Check sheet for the drawn part. Datum: minimum x, y, z corner. Units: mm. Coordinates: 2 decimals unless noted, no trailing zeros. Order: outer loops, then holes, each group sorted by start corner. A loop starts at its lowest first (then second) coordinate and runs counter-clockwise, first axis right, second up. Notation, with made-up numbers: M 62,66.5 L 94,66.5 A20 cw 94,105.5 Z; hole C 10,62 d11. An arc over 180 degrees is marked long. Return JSON: item names as keys, results as strings. Group by question number.
Q1. Section check C-C, the plane z = 1.1. Enter the section's corners in (x, y) (1 decimal), then the cut area to 3 significant figures.
Q2. Section check B-B, the plane x = 24.3. Count the separate pieces of the cut face and the enclosed holes in it, then the cut area to 3 significant figures.
Q3. Section check A-A, the plane y = 3. Enter the section's corners in (x, z).
Q4. Thickness scan on probe 1 along Y at (x, z) = (24.3, 0.3); probe 2 along X at (y, z) = (37.5, 0.5); probe 3 along X at (y, z) = (41.5, 1.25) (1 decimal). Record the ranges inside material, lowest first.
Q5. Section check D-D, the plane y = 40.31. Enter the section's corners in (x, z), then the cut area to 3 significant figures.
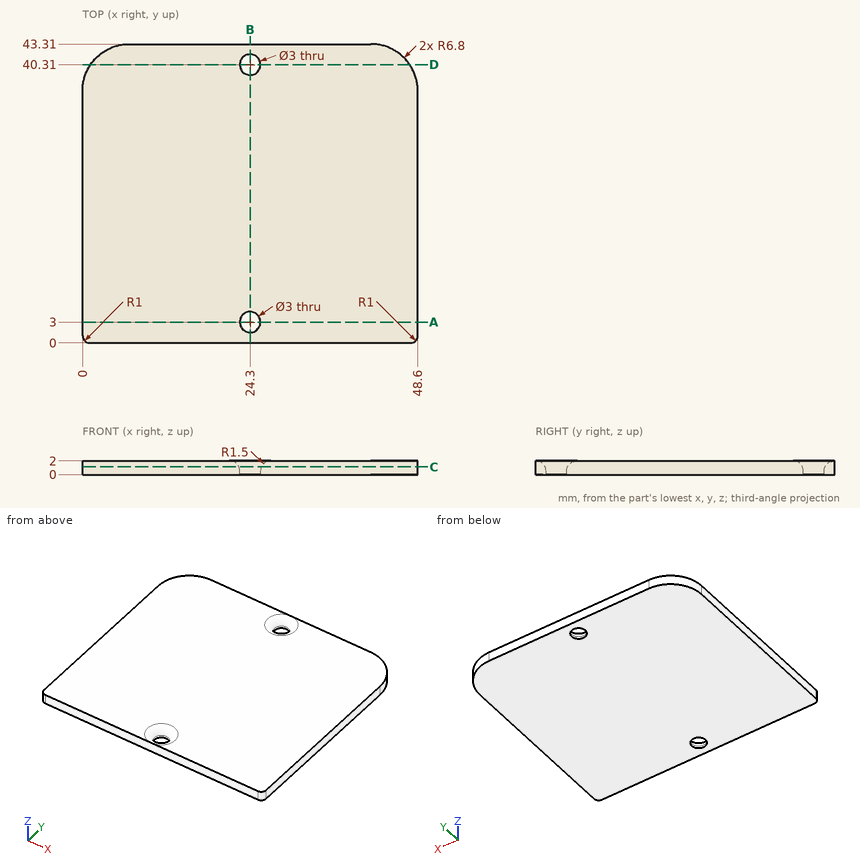
Numbers:
{
 "1": {"outline": "M 0,1 A1 ccw 1,0 L 47.6,0 A1 ccw 48.6,1 L 48.6,36.5 A6.8 ccw 41.8,43.3 L 6.8,43.3 A6.8 ccw 0,36.5 Z; hole C 24.3,3 d3.3; hole C 24.3,40.3 d3.3", "area": "2,070 mm2"},
 "2": {"separate pieces": "3", "enclosed holes": "0", "area": "72.7 mm2"},
 "3": {"outline": "M 0,0 L 22.8,0 L 22.8,0.5 A1.5 ccw 21.3,2 L 0,2 Z; M 25.8,0 L 48.6,0 L 48.6,2 L 27.3,2 A1.5 ccw 25.8,0.5 Z"},
 "4": {"probe 1": "y = 0 to 1.5, 4.5 to 38.81, 41.81 to 43.31", "probe 2": "x = 0.07 to 48.53", "probe 3": "x = 2.2 to 23.1, 25.5 to 46.4"},
 "5": {"outline": "M 1.16,0 L 22.8,0 L 22.8,0.5 A1.5 ccw 21.3,2 L 1.16,2 Z; M 25.8,0 L 47.44,0 L 47.44,2 L 27.3,2 A1.5 ccw 25.8,0.5 Z", "area": "85.6 mm2"}
}
